Design review of the part built by this model. Coordinates are the model's own, in mm. Face numbers are marked on the shaded views. A direction names the side the tool comes from. Give positions to 0.01 mm unless a question says otherwise; leave off trailing zeros. Write each loop counter-clockwise with the first axis right and the second up, starting at its lowest first coordinate (ties: lowest second). Pieces come first, ordered by that corner, then holes.
```python
from build123d import *

# Parameters (mm, degrees)
BOSS_EXTRUDE1_DEPTH     = 25.4
SKETCH4_R               = 3.302
CUT_EXTRUDE2_DEPTH      = 7.62
SKETCH2_R               = 3.175
SKETCH2_R_2             = 1.5875
CUT_EXTRUDE3_DEPTH      = 7.62
SKETCH6_W               = 128.1684
SKETCH6_H               = 12.7
BOSS_EXTRUDE2_DEPTH     = 7.62
SKETCH9_W               = 15.550542335
SKETCH9_H               = 50.8
BOSS_EXTRUDE3_DEPTH     = 7.62
CUT_EXTRUDE4_DEPTH      = 3.81
SKETCH10_R              = 2.921
CUT_EXTRUDE5_DEPTH      = 3.048
SKETCH11_R              = 1.5875
CUT_EXTRUDE6_DEPTH      = 106.41
CUT_EXTRUDE7_REACH      = 111.22
SKETCH12_W              = 8.89
SKETCH12_H              = 20.32
SKETCH13_R              = 3.175
BOSS_EXTRUDE4_DEPTH     = 7.62
CUT_EXTRUDE8_DEPTH      = 1
CUT_EXTRUDE8_DEPTH_BACK = 144.718942335


with BuildPart() as part:
    # Sketch1 → Boss-Extrude1 (new body)
    with BuildSketch(Plane(origin=(0, 0, 0), x_dir=(1, 0, 0), z_dir=(0, 1, 0))):
        Polygon((0, 0), (0, -101.6), (107.8484, -101.6), (107.8484, 0), (120.5484, 0), (120.5484, -109.22), (-7.62, -109.22), (-7.62, 0), align=None)
    extrude(amount=BOSS_EXTRUDE1_DEPTH)

    # Sketch4 → Cut-Extrude2 (cut)
    with BuildSketch(Plane.ZY.offset(-107.8484)):
        with Locations((25.4, 12.7)):
            Circle(SKETCH4_R)
    extrude(amount=-CUT_EXTRUDE2_DEPTH, mode=Mode.SUBTRACT)

    # Sketch2 → Cut-Extrude3 (cut)
    with BuildSketch(Plane(origin=(0, 0, 0), x_dir=(0, 0, -1), z_dir=(1, 0, 0))):
        with Locations((-25.4, 12.7)):
            Circle(SKETCH2_R)
        with Locations((-15.24, 12.7)):
            Circle(SKETCH2_R_2)
        with Locations((-35.56, 12.7)):
            Circle(SKETCH2_R_2)
    extrude(amount=-CUT_EXTRUDE3_DEPTH, mode=Mode.SUBTRACT)

    # Sketch6 → Boss-Extrude2 (add)
    with BuildSketch(Plane.XY.offset(109.22)):
        with Locations((56.4642, 31.75)):
            Rectangle(SKETCH6_W, SKETCH6_H)
        with Locations((56.4642, -6.35)):
            Rectangle(SKETCH6_W, SKETCH6_H)
    extrude(amount=-BOSS_EXTRUDE2_DEPTH)

    # Sketch9 → Boss-Extrude3 (add)
    with BuildSketch(Plane.XY.offset(109.22)):
        with Locations((128.323671168, 12.7)):
            Rectangle(SKETCH9_W, SKETCH9_H)
    extrude(amount=-BOSS_EXTRUDE3_DEPTH)

    # Sketch7 → Cut-Extrude4 (cut)
    with BuildSketch(Plane.XY.offset(109.22)):
        Polygon((40.910226472, 29.21), (38.527213236, 33.3375), (33.761186764, 33.3375), (31.378173528, 29.21), (33.761186764, 25.0825), (38.527213236, 25.0825), align=None)
        Polygon((132.350226472, -3.81), (129.967213236, 0.3175), (125.201186764, 0.3175), (122.818173528, -3.81), (125.201186764, -7.9375), (129.967213236, -7.9375), align=None)
    extrude(amount=-CUT_EXTRUDE4_DEPTH, mode=Mode.SUBTRACT)

    # Sketch10 → Cut-Extrude5 (cut)
    with BuildSketch(Plane.ZY.offset(7.62)):
        with Locations((15.24, 12.7)):
            Circle(SKETCH10_R)
        with Locations((35.56, 12.7)):
            Circle(SKETCH10_R)
    extrude(amount=-CUT_EXTRUDE5_DEPTH, mode=Mode.SUBTRACT)

    # Sketch11 → Cut-Extrude6 (cut, through all)
    with BuildSketch(Plane.XY.offset(105.41)):
        with Locations((36.1442, 29.21)):
            Circle(SKETCH11_R)
        with Locations((127.5842, -3.81)):
            Circle(SKETCH11_R)
    extrude(amount=-CUT_EXTRUDE6_DEPTH, mode=Mode.SUBTRACT)

    # Sketch12 → Cut-Extrude7 (cut, up to next)
    with BuildSketch(Plane.XY.offset(109.22), mode=Mode.PRIVATE) as cut_extrude7_sk1:
        with Locations((72.263, 12.7)):
            Rectangle(SKETCH12_W, SKETCH12_H)
    cut_extrude7_tool1 = extrude(cut_extrude7_sk1.sketch, amount=-CUT_EXTRUDE7_REACH, mode=Mode.PRIVATE) & part.part
    add(cut_extrude7_tool1.solids().sort_by_distance((72.263, 12.7, 109.22))[0], mode=Mode.SUBTRACT)

    # Sketch13 → Boss-Extrude4 (add)
    with BuildSketch(Plane.ZY.offset(7.62)):
        with Locations((25.4, 12.7)):
            Circle(SKETCH13_R)
    extrude(amount=-BOSS_EXTRUDE4_DEPTH)

    # Sketch14 → Cut-Extrude8 (cut, two sides)
    with BuildSketch(Plane.ZY.offset(7.62)) as cut_extrude8_sk:
        with BuildLine():
            Line((14.426351463, 25.4), (0, 25.4))
            Line((0, 25.4), (0, 0))
            Line((0, 0), (14.426351463, 0))
            ThreePointArc((14.426351463, 0), (6.276222595, 12.7), (14.426351463, 25.4))
        make_face()
    extrude(amount=CUT_EXTRUDE8_DEPTH, mode=Mode.SUBTRACT)
    extrude(cut_extrude8_sk.sketch, amount=-CUT_EXTRUDE8_DEPTH_BACK, mode=Mode.SUBTRACT)


solid = part.part
```
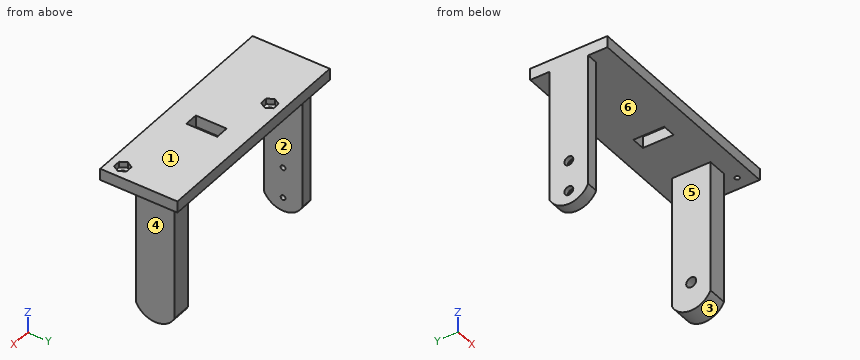
(1) Consider section C-C, the plane z = 25.4. Give the boundary of the cut face in (x, y).
Resolved:
outline: (-7.62, 0) - (0, 0) - (0, 25.4) - (-7.62, 25.4) - close; (107.85, 0) - (120.55, 0) - (120.55, 25.4) - (107.85, 25.4) - (107.85, 16) - (115.47, 16) - (115.47, 9.4) - (107.85, 9.4) - close
(2) Mouldability with a two-part tool opening along X and no side actions: class the marked faces 3, 4, 5 and 6 as pulls with the +X half, pulls with the -X half, needs draft (parallel to the pull), parting line crosses it, or undercut.
Resolved:
face 3: needs draft
face 4: pulls with the +X half
face 5: undercut
face 6: undercut
(3) Tool access review of the marked faces 1 and 2: name each direction out of +Z, -Z, +X, -X, +Y, -Y from which nothing blocks a thin tool from reaching the whole face with its end or side.
Resolved:
face 1: +Z, +X, -X, +Y, -Y
face 2: -Z, +Y, -Y
(4) To check wall thickness, follow L1, parallel to X at y = 25, z = 90.5; L2, parallel to Z at x = -5, y = 12; L3, parallel to Y at x = 109.5, z = 69. State the ranges of each line that lie inside material, in increasing order.
Resolved:
L1: x = -7.62 to 0, 107.85 to 120.55
L2: z = 6.29 to 12.4, 18.08 to 32.72, 38.4 to 109.22
L3: y = 0 to 25.4
(5) Consider section B-B, the plane y = 12.7. Give the number of separate pieces and of enclosed holes in the cut face, then the cut area to 3 significant figures.
Resolved:
separate pieces: 4
enclosed holes: 0
area: 2,850 mm2
(6) Consider section A-A, the plane z = 41. Give the boundary of the cut face in (x, y), then the cut area to 3 significant figures.
Resolved:
outline: (-7.62, 0) - (0, 0) - (0, 25.4) - (-7.62, 25.4) - close; (107.85, 0) - (120.55, 0) - (120.55, 25.4) - (107.85, 25.4) - close
area: 516 mm2
(7) Clearance check with flat-ended pins moving along their axes: P1, Ø5, axis at x = 92, y = 0.5, coming from the -Z side; P2, Ø8.5, axis at x = -2, z = 38, coming from the +Y side; P3, Ø12.5, axis at y = 17, z = 40, coming from the +X side; P4, Ø1, axis at y = -1.5, z = 96, coming from the -X side. State where each tip first meets the part, or that it passes through.
Resolved:
P1: stops at z = 101.6
P2: stops at y = 25.4
P3: stops at x = 120.55
P4: passes through
(8) Consider section D-D, the plane x = 24. Give the boundary of the cut face in (y, z), then the cut area to 3 significant figures.
Resolved:
outline: (-12.7, 101.6) - (38.1, 101.6) - (38.1, 109.22) - (-12.7, 109.22) - close
area: 387 mm2
